Model file for the job. Use its own axes, mm. A direction names the side the tool comes from. Coordinates: 2 decimals unless noted, no trailing zeros. Write each loop counter-clockwise with the first axis right and the second up, starting at its lowest first coordinate (ties: lowest second). Pieces come first, ordered by that corner, then holes. Notation, with made-up numbers: (51.25, -7) - (79.25, -7) arc R29 cw to (79.25, 22) - close; hole circle Ø1 at (56.25, 69.25). An arc over 180 degrees is marked (long way). Put each result on its own line as item: value. Start each with the question number.
1. Saw through at C-C, the plane y = -33. Write the cut outline in (x, z).
2. Pull direction Z, two halves, no side cores. Call faces 3 (the face through (142, -50, 69)), 4 (the face through (69, -39, 142)), 5 (the face through (69, -49, 0)), 6 (the face through (69, -49, 140)): released by +Z, released by -Z, zero draft, split by the parting line, or undercut.
3. Drop flat-ended pins along their axis: P1, Ø6, axis at x = 116.5, z = 89.5, coming from the +Y side; P2, Ø3, axis at x = 100.5, y = -77.5, coming from the -Z side. Give the stop position or say it passes through.
4. Drill centre lines: L1, parallel to Z at x = 134.5, y = -84; L2, parallel to Z at x = 70, y = -70. Where is each one in solid material? Low to high. Write a range as from..to.
5. Which spindle directions (+Z, -Z, +X, -X, +Y, -Y) get a long thin tool onto all of the face, cutting with end or side? Do faces 1 (the face through (71, -102, 69)), 2 (the face through (140, -49, 69)). Say none if no direction does.
6. Saw through at B-B, the plane x = 35.5. Write the cut outline in (y, z).
7. Saw through at D-D, the plane z = 123. Write the cut outline in (x, y).
8. Saw through at A-A, the plane y = -81.5. Write the cut outline in (x, z).
Autodesk Inventor part; units mm, degrees
ref_plane "YZ Plane" through (0, 0, 0) normal (1, 0, 0) x (0, 1, 0)
ref_plane "XZ Plane" through (0, 0, 0) normal (0, 1, 0) x (-1, 0, 0)
ref_plane "XY Plane" through (0, 0, 0) normal (0, 0, 1) x (1, 0, 0)
sketch "Sketch1" plane through (0, 0, 0) normal (0, 0, 1) x (1, 0, 0)
  line L0 (0, 0) -> (140, 0)
  line L1 (140, 0) -> (140, -100)
  line L2 (140, -100) -> (0, -100)
  line L3 (0, -100) -> (0, 0)
  dimension "d0" = 100
  dimension "d1" = 140
extrude "Extrusion1" add sketch "Sketch1" along normal blind 140
shell "Shell1" thickness 2 outward yes removed faces 1 at (93.3333, 0, 93.3333)
sketch "Sketch2" plane through (0, 0, 142) normal (0, 0, 1) x (1, 0, 0)
  line L0 (0, -100) -> (140, -100)
  line L1 (40, -50) -> (100, -50)
  line L2 (100, -50) -> (100, -100)
  line L3 (100, -100) -> (40, -100)
  line L4 (40, -100) -> (40, -50)
  line L5 (0, 0) -> (0, -100)
  line L6 (140, -100) -> (140, 0)
  line L7 (142, 0) -> (-2, 0)
  point P0 (40, -75)
  dimension "d5" = 40
  dimension "d6" = 40
  dimension "d7" = 50
extrude "Extrusion2" cut sketch "Sketch2" against normal blind 14 contours L4 L1 L2 L0
sketch "Sketch3" plane through (0, 0, -2) normal (0, 0, -1) x (-1, 0, 0)
  line L0 (-120, -72) -> (-20, -72)
  line L1 (-20, -72) -> (-20, -92)
  line L2 (-20, -92) -> (-120, -92)
  line L3 (-120, -92) -> (-120, -72)
  line L4 (0, 0) -> (0, -100)
  line L5 (-140, -100) -> (-140, 0)
  line L6 (2, -102) -> (-142, -102)
  point P0 (-120, -82)
  dimension "d13" = 20
  dimension "d14" = 20
  dimension "d15" = 20
  dimension "d16" = 10
extrude "Extrusion4" cut sketch "Sketch3" against normal blind 10
properties part number "Part2 Zaid"
Final values:
1. outline: (-2, -2) - (142, -2) - (142, 142) - (-2, 142) - close; hole (0, 0) - (140, 0) - (140, 140) - (0, 140) - close
2. face 3: zero draft
2. face 4: released by +Z
2. face 5: undercut
2. face 6: undercut
3. P1: stops at y = -100
3. P2: stops at z = 140
4. L1: z = -2..0, 140..142
4. L2: z = -2..0
5. face 1: +Z, -Z, +X, -X, -Y
5. face 2: +Y
6. outline: (-102, -2) - (-92, -2) - (-92, 0) - (-100, 0) - (-100, 140) - (0, 140) - (0, 142) - (-102, 142) - close; (-72, -2) - (0, -2) - (0, 0) - (-72, 0) - close
7. outline: (-2, -102) - (142, -102) - (142, 0) - (140, 0) - (140, -100) - (0, -100) - (0, 0) - (-2, 0) - close
8. outline: (-2, -2) - (20, -2) - (20, 0) - (0, 0) - (0, 140) - (40, 140) - (40, 142) - (-2, 142) - close; (100, 140) - (140, 140) - (140, 0) - (120, 0) - (120, -2) - (142, -2) - (142, 142) - (100, 142) - close
